Autodesk Fusion 360 part; units mm, degrees
sketch "Sketch7" plane through (0, 0, 0) normal (0, 0, 1) x (1, 0, 0)
  line L0 (0, 0) -> (108, 0)
  line L1 (0, 0) -> (0, 45)
  line L2 (0, 45) -> (108, 45)
  line L3 (108, 45) -> (108, 0)
  dimension "d135" = 108
  dimension "d136" = 45
extrude "Extrude7" add sketch "Sketch7" along normal blind 3
sketch "Sketch8" plane through (0, 0, 3) normal (0, 0, 1) x (-1, 0, 0)
  line L0 (0, 0) -> (-108, 0)
  line L1 (-108, 0) -> (-108, -45)
  line L2 (-108, -45) -> (0, -45)
  line L3 (0, -45) -> (0, 0)
  circle A0 centre (-5, -35) radius 2
  circle A1 centre (-5, -10) radius 2
  circle A2 centre (-11, -35) radius 2
  circle A3 centre (-17, -35) radius 2
  circle A4 centre (-11, -10) radius 2
  circle A5 centre (-17, -10) radius 2
  circle A6 centre (-46.5, -22.5) radius 2
  circle A7 centre (-103, -35) radius 2
  circle A8 centre (-103, -10) radius 2
  circle A9 centre (-97, -10) radius 2
  circle A10 centre (-91, -10) radius 2
  circle A11 centre (-91, -35) radius 2
  circle A12 centre (-97, -35) radius 2
  circle A13 centre (-61.5, -22.5) radius 2
  dimension "d142" = 6
  dimension "d143" = 6
  dimension "d144" = 6
  dimension "d145" = 6
  dimension "d146" = 4
  dimension "d147" = 4
  dimension "d148" = 4
  dimension "d149" = 4
  dimension "d150" = 4
  dimension "d151" = 4
  dimension "d153" = 4
extrude "Extrude8" cut sketch "Sketch8" against normal blind 3 contours A0 | A1 | A2 | A3 | A4 | A5 | A6 | A7 | A8 | A9 | A10 | A11 | A12 | A13
fillet "Fillet13" radius 1 1 edges at (54, 0, 3)
fillet "Fillet14" radius 1 1 edges at (54, 0, 0)
fillet "Fillet15" radius 1 1 edges at (54, 45, 3)
fillet "Fillet16" radius 1 1 edges at (54, 45, 0)
The model under review builds one solid part; all positions refer to its coordinate system, in mm. Round coordinates to 2 decimals unless told otherwise and drop trailing zeros. Loops run counter-clockwise (first coordinate to the right, second up) from the corner with the lowest first, then second, coordinate; pieces in that order, holes last. Notation, with made-up numbers: (-20, -34) -> (12, -34) arc R29 ccw to (12, -5) -> close; hole circle Ø4 at (0, -5). An arc over 180 degrees is marked (long way). Answer as CSV lines item,"result".
1) Add section C-C on x = 11. Write out the cut boundary in (y, z), plus the area to 3 significant figures.
Geometry results:
outline,"(0, 1) arc R1 ccw to (1, 0) -> (8, 0) -> (8, 3) -> (1, 3) arc R1 ccw to (0, 2) -> close; (12, 0) -> (33, 0) -> (33, 3) -> (12, 3) -> close; (37, 0) -> (44, 0) arc R1 ccw to (45, 1) -> (45, 2) arc R1 ccw to (44, 3) -> (37, 3) -> close"
area,"110 mm²"
2) Draft analysis for pull direction X (two halves, no side actions). For faces 1 (the face through (108, 23, 1)), 2 (the face through (12.474, 8.648, 1.521)), 3 (the face through (53, 23, 3)), 4 (the face through (11, 37, 2)), state which applies: pulls with the +X half, pulls with the -X half, needs draft (parallel to the pull), parting line crosses it, or undercut.
Geometry results:
face 1,"pulls with the +X half"
face 2,"undercut"
face 3,"needs draft"
face 4,"undercut"
3) To check wall thickness, follow line 1 along Y through (x, z) = (5, 1.1); line 2 along X through (y, z) = (22.5, 2.35); line 3 along Y through (x, z) = (103, 0.6). State the ranges of each line that lie inside material, in increasing order. Write a range as from..to.
Geometry results:
line 1,"y = 0..8, 12..33, 37..45"
line 2,"x = 0..44.5, 48.5..59.5, 63.5..108"
line 3,"y = 0.08..8, 12..33, 37..44.92"
4) For P1, Ø1.5, axis at x = 66, z = 1, coming from the -Y side, flat-tipped, find the tip position at first contact; note if it passes through.
Geometry results:
P1,"stops at y = 0"
5) Add section A-A on y = 10. Write out the cut boundary in (x, z).
Geometry results:
outline,"(0, 0) -> (3, 0) -> (3, 3) -> (0, 3) -> close; (7, 0) -> (9, 0) -> (9, 3) -> (7, 3) -> close; (13, 0) -> (15, 0) -> (15, 3) -> (13, 3) -> close; (19, 0) -> (89, 0) -> (89, 3) -> (19, 3) -> close; (93, 0) -> (95, 0) -> (95, 3) -> (93, 3) -> close; (99, 0) -> (101, 0) -> (101, 3) -> (99, 3) -> close; (105, 0) -> (108, 0) -> (108, 3) -> (105, 3) -> close"
6) Add section D-D on z = 0.45. State how many separate pieces and enclosed holes the cut face has, plus the area to 3 significant figures.
Geometry results:
separate pieces,"1"
enclosed holes,"14"
area,"4,650 mm²"
7) Add section B-B on x = 61.5. Write out the cut boundary in (y, z), plus the area to 3 significant figures.
Geometry results:
outline,"(0, 1) arc R1 ccw to (1, 0) -> (20.5, 0) -> (20.5, 3) -> (1, 3) arc R1 ccw to (0, 2) -> close; (24.5, 0) -> (44, 0) arc R1 ccw to (45, 1) -> (45, 2) arc R1 ccw to (44, 3) -> (24.5, 3) -> close"
area,"122 mm²"
